Could you check a few things on this model? Use its own coordinates, in mm. A direction names the side the tool comes from. Give positions to 0.01 mm unless a question says otherwise; leave off trailing zeros. Write each loop counter-clockwise with the first axis right and the second up, starting at its lowest first coordinate (ties: lowest second). Pieces come first, ordered by that corner, then holes. Notation, with made-up numbers: M -0.5,63 L 28.5,63 A9 cw 28.5,76 Z; hole C -32.75,86.25 d11. An arc over 180 degrees is marked long. One line per item, written item: value.
```python
from build123d import *

# Parameters (mm, degrees)
F1_DEPTH = 7.62
F2_DEPTH = 7.62
F0_W     = 35.56
F0_H     = 6.35
F0_W_2   = 8.89
F0_H_2   = 2.54
F3_DEPTH = 5.08
F4_DEPTH = 5.08
F6_DEPTH = 44.45


with BuildPart() as f1:
    # F0 (on Front) → F1 (new body)
    with BuildSketch(Plane.XZ):
        Polygon((34.29, 8.89), (34.29, 0), (57.15, 0), (57.15, 6.35), (57.15, 8.89), align=None)
    extrude(amount=F1_DEPTH)

    # F0 (on Front) → F2 (join)
    with BuildSketch(Plane.XZ):
        Polygon((34.29, 8.89), (34.29, 0), (57.15, 0), (57.15, 6.35), (57.15, 8.89), align=None)
    extrude(amount=-F2_DEPTH)

    # F0 (on Front) → F3 (join)
    with BuildSketch(Plane.XZ):
        with Locations((74.93, 3.175)):
            Rectangle(F0_W, F0_H)
        with Locations((97.155, 3.175)):
            Rectangle(F0_W_2, F0_H)
        with Locations((97.155, -1.27)):
            Rectangle(F0_W_2, F0_H_2)
    extrude(amount=F3_DEPTH)

    # F0 (on Front) → F4 (join)
    with BuildSketch(Plane.XZ):
        with Locations((74.93, 3.175)):
            Rectangle(F0_W, F0_H)
        with Locations((97.155, 3.175)):
            Rectangle(F0_W_2, F0_H)
        with Locations((97.155, -1.27)):
            Rectangle(F0_W_2, F0_H_2)
    extrude(amount=-F4_DEPTH)

    # F5 (on face) → F6 (join)
    with BuildSketch(Plane.YZ.offset(101.6)):
        Polygon((0, 10.16), (0, 6.35), (5.08, 6.35), align=None)
        Polygon((-5.08, 6.35), (0, 6.35), (0, 10.16), align=None)
    extrude(amount=-F6_DEPTH)


solid = f1.part
```
1) If we section it at C-C, the plane z = 5.25: Write out the boundary of the cut face in (x, y), then the cut area to 3 significant figures.
Outcome:
outline: M 34.29,-7.62 L 57.15,-7.62 L 57.15,-5.08 L 101.6,-5.08 L 101.6,5.08 L 57.15,5.08 L 57.15,7.62 L 34.29,7.62 Z
area: 800 mm^2
2) If we section it at D-D, the plane x = 95: Write out the boundary of the cut face in (y, z), then the cut area to 3 significant figures.
Outcome:
outline: M -5.08,-2.54 L 5.08,-2.54 L 5.08,6.35 L 0,10.16 L -5.08,6.35 Z
area: 110 mm^2
3) Please list where these lines run through material, in increasing order: L1, parallel to X at y = 6.75, z = 6.5; L2, parallel to Y at x = 75.5, z = 1.25; L3, parallel to X at y = -1, z = -1. Write a range as from..to.
Outcome:
L1: x = 34.29..57.15
L2: y = -5.08..5.08
L3: x = 92.71..101.6
4) If we section it at A-A, the plane x = 84: Write out the boundary of the cut face in (y, z), then the cut area to 3 significant figures.
Outcome:
outline: M -5.08,0 L 5.08,0 L 5.08,6.35 L 0,10.16 L -5.08,6.35 Z
area: 83.9 mm^2
5) I'm going to push flat-ended pins straight in: pin 1 (4.5 mm diameter, centred on x = 49, y = -0.5, fed in from +Z); pin 2 (4 mm diameter, centred on x = 72.5, z = -1, fed in from -Y); pin 3 (1 mm diameter, centred on y = 0, z = 9.5, fed in from -X). Where does each tip first touch, or does it pass through?
Outcome:
pin 1: stops at z = 8.89
pin 2: stops at y = -5.08
pin 3: stops at x = 57.15
6) On a 3-axis mill with a long thin cutter (end or side, diameter ignored), from which of +Z, -Z, +X, -X, +Y, -Y can I reach the whole of each face in a straight line? I mean faces 1 (the face through (79, 5.08, 3)), 2 (the face through (57.15, 6, 5)), 3 (the face through (63, 0, 0)), 4 (the face through (46, 0, 8.89)), 5 (the face through (79.686, -2.504, 8.282)). Say none if no direction works.
Outcome:
face 1: +Z, -Z, +X, +Y
face 2: +Z, +X, +Y
face 3: -Z, -X, +Y, -Y
face 4: +Z, -X, +Y, -Y
face 5: +Z, +X, -Y
7) If we section it at B-B, the plane y = -1: Write out the boundary of the cut face in (x, z).
Outcome:
outline: M 34.29,0 L 92.71,0 L 92.71,-2.54 L 101.6,-2.54 L 101.6,9.41 L 57.15,9.41 L 57.15,8.89 L 34.29,8.89 Z
